CAD build for the part. Positions are in the model's coordinates, mm. A direction names the side the tool comes from. Round coordinates to 2 decimals unless told otherwise and drop trailing zeros. Write each loop counter-clockwise with the first axis right and the second up, starting at its lowest first coordinate (ties: lowest second). Pieces come first, ordered by that corner, then holes. Notation, with made-up numbers: (71, 73) -> (103, 73) arc R26 cw to (103, 94) -> close; hole circle Ø2 at (-11, 34.5). An arc over 180 degrees is marked (long way). Put each result on its own line as item: value. Start each with the question number.
1. Drill centre lines: line 1 (X direction, y = 8, z = 0); line 2 (Z direction, x = -6, y = 7.5); line 3 (X direction, y = 8.5, z = -1.25). Where is each one in solid material? Low to high. Write a range as from..to.
2. Pull direction Z, two halves, no side cores. Call faces 5 (the flat face through (-6.06, 4.93, 1.01)), 6 (the flat face through (2.89, 4.93, -5.48)), 7 (the flat face through (2.906, 4.93, 5.342)): pulls with the +Z half, pulls with the -Z half, needs draft (parallel to the pull), parting line crosses it, or undercut.
3. Saw through at B-B on x = 2.5. List the corners of the cut face in (y, z), and give its area (3 significant figures).
4. 3-axis set-ups, long thin cutter, end or side, ignore diameter. For faces 1 (the flat face through (0.826, 4.93, -6.177)), 2 (the flat face through (-6.03, 4.93, -1.16)), 3 (the flat face through (-2.9, 4.93, 5.32)), 4 (the flat face through (6.05, 4.93, -1.17)): which of +Z, -Z, +X, -X, +Y, -Y reach the whole face in a straight line?
5. Saw through at C-C on z = 3. List the corners of the cut face in (x, y).
6. Saw through at A-A on z = 0.5. List the corners of the cut face in (x, y).
7. Flat gauge pins, fed straight in: P1, Ø1.5, axis at x = 5.5, y = 3, coming from the +Z side; P2, Ø1.5, axis at y = 7, z = -0.5, coming from the -X side. Where does each tip first touch, or does it go through?
from build123d import *

# Parameters (mm, degrees)
SKETCH2_R           = 2
BOSS_EXTRUDE1_DEPTH = 10
FILLET1_R           = 0.3


with BuildPart() as part:
    # Sketch2 → Boss-Extrude1 (new body)
    with BuildSketch(Plane(origin=(0, 0, 0), x_dir=(1, 0, 0), z_dir=(0, 1, 0))):
        Polygon((-0.35, 7.485859039), (0.35, 7.485859039), (1.242069669, 5.034917766), (1.906773221, 4.815442965), (4.069099878, 6.273950712), (4.635411774, 5.862501035), (3.916484162, 3.355302497), (4.325236581, 2.787040708), (6.931884937, 2.696014542), (7.148196833, 2.03027498), (5.092877853, 0.424483803), (5.089549606, -0.275508285), (7.144868587, -1.881299462), (6.928556691, -2.547039024), (4.321908334, -2.63806519), (3.907770701, -3.202414391), (4.626698313, -5.709612929), (4.060386417, -6.121062606), (1.898059759, -4.662554859), (1.231299238, -4.87569896), (0.339229569, -7.326640233), (-0.360770431, -7.326640233), (-1.2528401, -4.87569896), (-1.917543652, -4.656224159), (-4.079870309, -6.114731905), (-4.646182205, -5.703282228), (-3.927254593, -3.196083691), (-4.336007012, -2.627821902), (-6.942655368, -2.536795735), (-7.158967264, -1.871056174), (-5.103648284, -0.265264996), (-5.100320037, 0.434727091), (-7.155639018, 2.040518269), (-6.939327122, 2.70625783), (-4.332678765, 2.797283997), (-3.918541132, 3.361633198), (-4.637468744, 5.868831735), (-4.071156848, 6.280281412), (-1.90883019, 4.821773666), (-1.242069669, 5.034917766), align=None)
        with Locations(Location((0, 0, 0), (0, 0, 270))):
            Circle(SKETCH2_R, mode=Mode.SUBTRACT)
    extrude(amount=BOSS_EXTRUDE1_DEPTH)

    # Fillet1
    fillet1_edges = [part.edges().sort_by_distance(p)[0] for p in [
        (-0.35, 5, -7.485859039),
        (0.35, 5, -7.485859039),
        (4.069099878, 5, -6.273950712),
        (4.635411774, 5, -5.862501035),
        (6.931884937, 5, -2.696014542),
        (7.148196833, 5, -2.03027498),
        (7.144868587, 5, 1.881299462),
        (6.928556691, 5, 2.547039024),
        (4.626698313, 5, 5.709612929),
        (4.060386417, 5, 6.121062606),
        (0.339229569, 5, 7.326640233),
        (-0.360770431, 5, 7.326640233),
        (-4.079870309, 5, 6.114731905),
        (-4.646182205, 5, 5.703282228),
        (-6.942655368, 5, 2.536795735),
        (-7.158967264, 5, 1.871056174),
        (-7.155639018, 5, -2.040518269),
        (-6.939327122, 5, -2.70625783),
        (-4.637468744, 5, -5.868831735),
        (-4.071156848, 5, -6.280281412),
    ]]
    fillet(fillet1_edges, radius=FILLET1_R)


solid = part.part
Return value:
1. line 1: x = -5.1..-2, 2..5.09
1. line 2: z = -2.74..-1.14, 0.97..2.57
1. line 3: x = -6.14..-1.56, 1.56..6.15
2. face 5: undercut
2. face 6: pulls with the -Z half
2. face 7: pulls with the +Z half
3. outline: (0, -5.22) -> (10, -5.22) -> (10, 5.07) -> (0, 5.07) -> close
3. area: 103 mm^2
4. face 1: -Z, +Y, -Y
4. face 2: -X, +Y, -Y
4. face 3: +Z, +Y, -Y
4. face 4: +X, +Y, -Y
5. outline: (-4.07, 0) -> (4.06, 0) -> (4.06, 10) -> (-4.07, 10) -> close
6. outline: (-5.4, 0) -> (-1.94, 0) -> (-1.94, 10) -> (-5.4, 10) -> close; (1.94, 0) -> (5.38, 0) -> (5.38, 10) -> (1.94, 10) -> close
7. P1: stops at z = 2.62
7. P2: stops at x = -6.14
